Can you work these out from the model? Positions are in its coordinate system, mm. A direction names the side the tool comes from. Coordinates: 2 decimals unless noted, no trailing zeros. Order: outer loops, then holes, each group sorted by start corner. A loop starts at its lowest first (then second) coordinate and runs counter-clockwise, first axis right, second up. Notation, with made-up numbers: (3, 2) - (29, 2) arc R30 cw to (29, 38) - close; hole circle Ø9 at (-39, -40). An arc over 180 degrees is marked (long way). Return JSON: item names as keys, results as strings. Group by question number.
1) Imagine slicing it at C-C (x = -6.5). Write out the boundary of the cut face in (y, z), and give its area (3 significant figures).
2) If I drill on line 1 along X through (y, z) = (-30, -2.5); line 2 along X through (y, z) = (5, -2); line 3 along Y through (x, z) = (9.5, 29.5), over which ranges is the centre line in solid material (lowest first)?
3) Imagine slicing it at A-A (y = 0). Write out the boundary of the cut face in (x, z).
4) Imagine slicing it at B-B (z = 0). Write out the boundary of the cut face in (x, y), and give its area (3 significant figures).
5) For pin 1 Ø4 at (x, z) = (4.5, 23) entering from -Y; pin 2 Ø12 at (x, z) = (9, -18) entering from -Y; pin 3 Ø5 at (x, y) = (8.5, -28) entering from -Z, each with a flat end and sliding along its axis, tell me the tip position at first contact or that it passes through.
6) Imagine slicing it at D-D (x = 27.5). Write out the boundary of the cut face in (y, z), and give its area (3 significant figures).
7) Which directions (+Z, -Z, +X, -X, +Y, -Y) give clear straight access to the entire face, cutting with the end or side of a thin tool? Please do faces 1 (the face through (-30, 31, 0)), 2 (the face through (10, -11, 11)), 3 (the face through (-19.86, 24.383, -2.103)).
```python
from build123d import *

# Parameters (mm, degrees)
F0_R     = 45
F0_R_2   = 15
F1_DEPTH = 10
F2_DEPTH = 60
F3_DEPTH = 30


with BuildPart() as f1:
    # F0 (on Right) → F1 (new body, symmetric)
    with BuildSketch(Plane.YZ):
        Circle(F0_R)
        Circle(F0_R_2, mode=Mode.SUBTRACT)
        with BuildLine():
            ThreePointArc((38.06, 0), (31.06, -7), (24.06, 0))
            ThreePointArc((24.06, 0), (31.06, 7), (38.06, 0))
        make_face(mode=Mode.SUBTRACT)
        Circle(F0_R_2)
        with BuildLine():
            ThreePointArc((38.06, 0), (31.06, 7), (24.06, 0))
            ThreePointArc((24.06, 0), (31.06, -7), (38.06, 0))
        make_face()
    extrude(amount=F1_DEPTH, both=True)

    # F0 (on Right) → F2 (join)
    with BuildSketch(Plane.YZ):
        Circle(F0_R_2)
    extrude(amount=F2_DEPTH)

    # F0 (on Right) → F3 (join)
    with BuildSketch(Plane.YZ):
        with BuildLine():
            ThreePointArc((38.06, 0), (31.06, 7), (24.06, 0))
            ThreePointArc((24.06, 0), (31.06, -7), (38.06, 0))
        make_face()
    extrude(amount=-F3_DEPTH)


solid = f1.part
```
Calculated:
{
 "1": {"outline": "circle Ø90 at (0, 0)", "area": "6,360 mm2"},
 "2": {"line 1": "-10 to 10", "line 2": "-10 to 60", "line 3": "-33.98 to 33.98"},
 "3": {"outline": "(-10, -45) - (10, -45) - (10, -15) - (60, -15) - (60, 15) - (10, 15) - (10, 45) - (-10, 45) - close"},
 "4": {"outline": "(-30, 24.06) - (-10, 24.06) - (-10, -45) - (10, -45) - (10, -15) - (60, -15) - (60, 15) - (10, 15) - (10, 45) - (-10, 45) - (-10, 38.06) - (-30, 38.06) - close", "area": "3,580 mm2"},
 "5": {"pin 1": "y = -39.8", "pin 2": "y = -43.37", "pin 3": "z = -37.08"},
 "6": {"outline": "circle Ø30 at (0, 0)", "area": "707 mm2"},
 "7": {"face 1": "+Z, -Z, -X, +Y, -Y", "face 2": "+X", "face 3": "-X"}
}
